Study the drawing (mm; zero at the part's minimum x, y, z) and answer. A direction names the side the tool comes from. Coordinates: 2 decimals unless noted, no trailing zeros. Order: outer loops, then holes, each group sorted by start corner. A loop starts at its lowest first (then second) coordinate and runs counter-clockwise, first axis right, second up. Notation, with made-up numbers: (64, -32.5) -> (109, -32.5) arc R16 cw to (109, -20.5) -> close; hole circle Ø5 at (70.5, 70). An arc over 180 degrees is marked (long way). Answer as CSV lines item,"result". Start each with the question number.
Item 1: Which of the six approach directions +Z, -Z, +X, -X, +Y, -Y give full straight-line access (tool end or side, diameter ignored) to the marked faces 1, 2 and 3?
Item 2: Section B-B (z = 22) is taken. Write down the section's boundary in (x, y).
Item 3: Straight lines are drawn through the part: L1, parallel to Z at x = 11, y = 28.5; L2, parallel to X at y = 10.25, z = 28; L3, parallel to Y at x = 8, z = 4. For each, find the intervals that lie inside material, in ascending order.
Item 4: Section D-D (x = 34) is taken. Write down the section's boundary in (y, z), then the cut area to 3 significant figures.
Item 5: Each of these flat-tipped pins is pushed along its axis until it touches: pin 1 Ø1.5 at (x, y) = (10, 25.5) entering from -Z; pin 2 Ø4 at (x, z) = (15, 12) entering from +Y; pin 3 Ø10 at (y, z) = (23.5, 29.5) entering from +X. Where does it stop, or does it pass through?
Item 6: Section C-C (y = 24.5) is taken. Write down the section's boundary in (x, z), then the cut area to 3 significant figures.
Item 7: Section A-A (x = 8) is taken. Write down the section's boundary in (y, z), then the cut area to 3 significant figures.
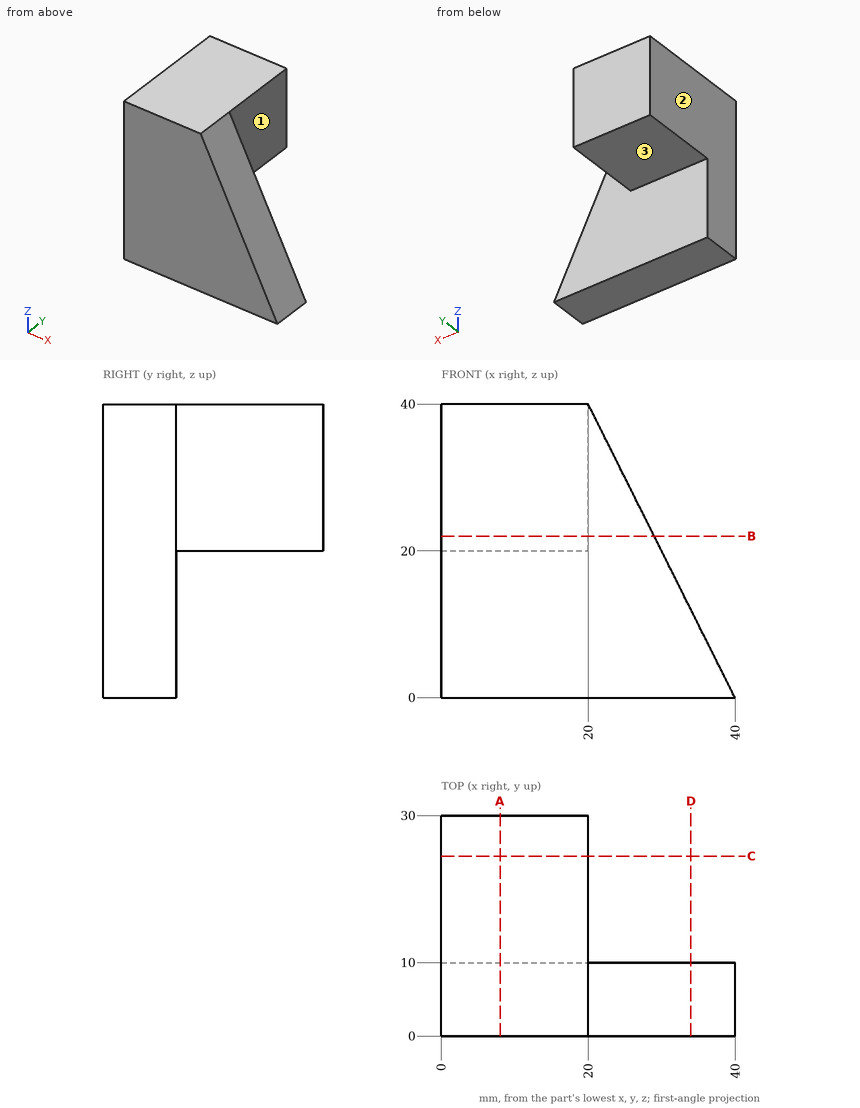
Checked values:
1,face 1,"+Z, -Z, +X, +Y"
1,face 2,"+Z, -Z, -X, +Y, -Y"
1,face 3,"-Z, +X, -X, +Y"
2,outline,"(0, 0) -> (29, 0) -> (29, 10) -> (20, 10) -> (20, 30) -> (0, 30) -> close"
3,L1,"z = 20 to 40"
3,L2,"x = 0 to 20"
3,L3,"y = 0 to 10"
4,outline,"(0, 0) -> (10, 0) -> (10, 12) -> (0, 12) -> close"
4,area,"120 mm^2"
5,pin 1,"stops at z = 20"
5,pin 2,"stops at y = 10"
5,pin 3,"stops at x = 20"
6,outline,"(0, 20) -> (20, 20) -> (20, 40) -> (0, 40) -> close"
6,area,"400 mm^2"
7,outline,"(0, 0) -> (10, 0) -> (10, 20) -> (30, 20) -> (30, 40) -> (0, 40) -> close"
7,area,"800 mm^2"
